Geometry: final body of the model. Coordinates: model frame, mm. Face numbers are marked on the shaded views. Give positions to 0.01 mm unless a question says otherwise; leave off trailing zeros. Loops run counter-clockwise (first coordinate to the right, second up) from the corner with the lowest first, then second, coordinate; pieces in that order, holes last.
```python
from build123d import *

# Parameters (mm, degrees)
F2_R     = 88.9
F0_R     = 59.26709
F4_T     = -6.35
F5_R     = 54.9232413826
F6_DEPTH = 6.3510001
F7_R     = 3.17499


# Not quite as in the source:
# - a fillet or chamfer is up to 0.001 mm smaller than in the source, because OpenCascade refuses the exact size


with BuildPart() as f3:
    # F2 (on offset) → F3 section 0
    with BuildSketch(Plane.XZ.offset(76.2)):
        Circle(F2_R)
    # F0 (on Front) → F3 section 1
    with BuildSketch(Plane.XZ):
        Circle(F0_R)
    loft()

    # F4
    f4_openings = [f3.faces().sort_by_distance(p)[0] for p in [
        (0, -76.2, 0),
    ]]
    offset(amount=F4_T, openings=f4_openings, kind=Kind.INTERSECTION)

    # F5 (on face) → F6 (cut, through all)
    with BuildSketch(Plane.XZ.offset(6.35)):
        Circle(F5_R)
    extrude(amount=-F6_DEPTH, mode=Mode.SUBTRACT)

    # F7 (radius 3.175 in the source; OpenCascade refuses exactly that, so slightly less here)
    f7_edges = [f3.edges().sort_by_distance(p)[0] for p in [
        (-88.9, -76.2, 0),
        (-82.086742, -76.2, 0),
    ]]
    fillet(f7_edges, radius=F7_R)

    # F8 (on Top) → F9 (revolve, cut)
    with BuildSketch(Plane.XY):
        with BuildLine():
            Line((0, 0), (-59.26709, 0))
            ThreePointArc((-59.26709, 0), (-30.7694079322, -12.346744825), (0, -16.5661673578))
            Line((0, -16.5661673578), (0, 0))
        make_face()
    revolve(axis=Axis((0, -8.2830836789, 0), (0, -1, 0)), mode=Mode.SUBTRACT)


solid = f3.part
```
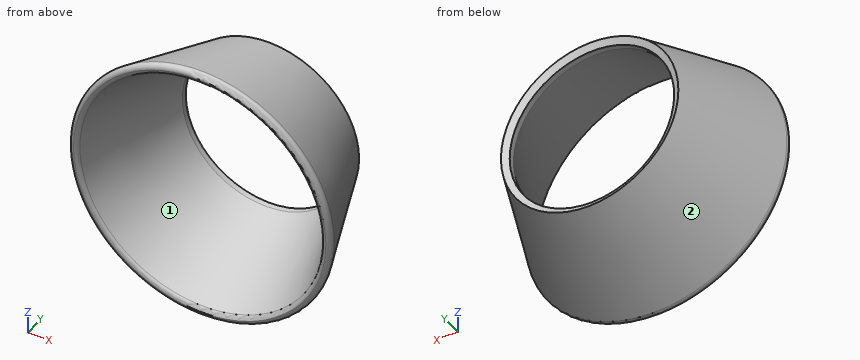
Q1. Section query C-C, the plane y = -47. Return loops of the section in (x, z).
Q2. Pin query (flat end, axial travel): pin 1 Ø3 at (y, z) = (-20.5, 42) entering from +X; pin 2 Ø10 at (y, z) = (-28, -26) entering from +X; pin 3 Ø4 at (y, z) = (-24, -20) entering from -X. Return the tip coordinate at first contact, or that it passes through.
Q3. Mould query, pull axis X, two halves, no side actions, for the marked faces 1 and 2. Classes: +X half, -X half, draft (parallel to the pull), parting line (faces both ways), or undercut.
Q4. Material intervals for probe 1 along Z at (x, y) = (-42, -5.5); probe 2 along Z at (x, y) = (40, -17.5); probe 3 along X at (y, z) = (-17, -48), sorted ascending.
Q5. Section query B-B, the plane y = -68.5. Return loops of the section in (x, z).
Resolved:
1. outline: circle Ø155.09 at (0, 0); hole circle Ø141.46 at (0, 0)
2. pin 1: stops at x = 53.89
2. pin 2: stops at x = 67.93
2. pin 3: stops at x = -66.62
3. face 1: undercut
3. face 2: parting line
4. probe 1: z = -44.8 to -35.39, 35.39 to 44.8
4. probe 2: z = -52.59 to -43.72, 43.72 to 52.59
4. probe 3: x = -45.12 to -34.42, 34.42 to 45.12
5. outline: circle Ø171.81 at (0, 0); hole circle Ø158.18 at (0, 0)
